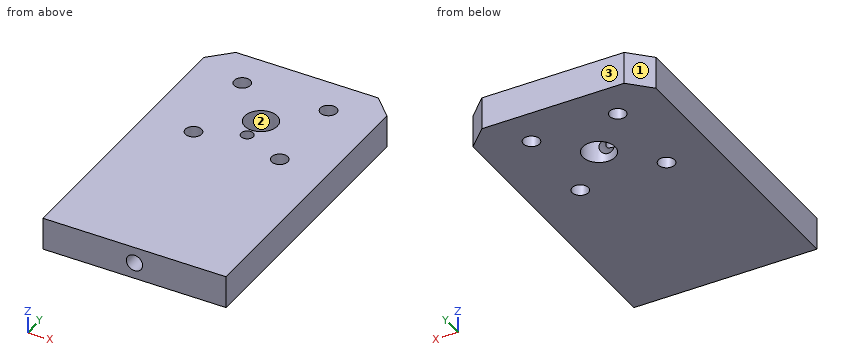
```python
from build123d import *

# Parameters (mm, degrees)
F0_R     = 2
F0_R_2   = 4
F1_DEPTH = 8
F2_R     = 2
F3_DEPTH = 53
F4_R     = 1.5
F5_DEPTH = 3


with BuildPart() as f1:
    # F0 (on Top) → F1 (new body)
    with BuildSketch(Plane.XY):
        Polygon((0, 70), (0, 0), (45, 0), (45, 70), (40, 75), (5, 75), align=None)
        with Locations((11.893398, 44.393398)):
            Circle(F0_R, mode=Mode.SUBTRACT)
        with Locations((11.893398, 65.606602)):
            Circle(F0_R, mode=Mode.SUBTRACT)
        with Locations((33.106602, 44.393398)):
            Circle(F0_R, mode=Mode.SUBTRACT)
        with Locations((22.5, 55)):
            Circle(F0_R_2, mode=Mode.SUBTRACT)
        with Locations((33.106602, 65.606602)):
            Circle(F0_R, mode=Mode.SUBTRACT)
    extrude(amount=F1_DEPTH)

    # F2 (on face) → F3 (cut)
    with BuildSketch(Plane.XZ):
        with Locations((22.5, 4)):
            Circle(F2_R)
    extrude(amount=-F3_DEPTH, mode=Mode.SUBTRACT)

    # F4 (on face) → F5 (cut)
    with BuildSketch(Plane.XY.offset(8)):
        with Locations((22.5, 49)):
            Circle(F4_R)
    extrude(amount=-F5_DEPTH, mode=Mode.SUBTRACT)


solid = f1.part
```
Work out the finished part from the listing and answer in its coordinate system (mm). Face numbers are marked on the shaded views. Give positions to 0.01 mm unless a question says otherwise; leave off trailing zeros. Loops run counter-clockwise (first coordinate to the right, second up) from the corner with the lowest first, then second, coordinate; pieces in that order, holes last. Notation, with made-up numbers: (41, -25.75) -> (74, -25.75) arc R21 cw to (74, 0.25) -> close; hole circle Ø4 at (-30.5, 34). An arc over 180 degrees is marked (long way). One line per question, with ' | ' between items. Start each with the question number.
1) Section B-B, the plane y = 32.5 is taken. Determine the outline of the cut face in (x, z).
2) Straight lines are drawn through the part: L1, parallel to Y at x = 33, z = 7.5; L2, parallel to Z at x = 22.5, y = 38.5; L3, parallel to X at y = 65, z = 2.5. For each, find the intervals that lie inside material, in ascending order.
3) This flat-tipped pin is pushed along its axis until it touches: pin 1 (3.5 mm diameter, centred on x = 33.11, y = 44.39, fed in from -Z). Where does it stop, or does it pass through?
4) Section A-A, the plane x = 22.5 is taken. Determine the outline of the cut face in (y, z), then the cut area to 3 significant figures.
5) Section C-C, the plane y = 55 is taken. Determine the outline of the cut face in (x, z), then the cut area to 3 significant figures.
6) Determine the mould class of the marked faces 1, 2 and 3 for opening direction X: +X half, -X half, draft (parallel to the pull), parting line (faces both ways), or undercut.
7) Section D-D, the plane z = 4 is taken. Determine the outline of the cut face in (x, y).
Resolved:
1) outline: (0, 0) -> (45, 0) -> (45, 8) -> (0, 8) -> close; hole circle Ø4 at (22.5, 4)
2) L1: 0 to 42.4, 46.39 to 63.61, 67.6 to 75 | L2: 0 to 2, 6 to 8 | L3: 0 to 9.99, 13.8 to 31.2, 35.01 to 45
3) pin 1: through
4) outline: (0, 0) -> (51, 0) -> (51, 2) -> (0, 2) -> close; (0, 6) -> (47.5, 6) -> (47.5, 8) -> (0, 8) -> close; (50.5, 6) -> (51, 6) -> (51, 8) -> (50.5, 8) -> close; (59, 0) -> (75, 0) -> (75, 8) -> (59, 8) -> close | area: 326 mm2
5) outline: (0, 0) -> (18.5, 0) -> (18.5, 8) -> (0, 8) -> close; (26.5, 0) -> (45, 0) -> (45, 8) -> (26.5, 8) -> close | area: 296 mm2
6) face 1: -X half | face 2: undercut | face 3: draft
7) outline: (0, 0) -> (20.5, 0) -> (20.5, 51.54) arc R4 cw (long way) to (24.5, 51.54) -> (24.5, 0) -> (45, 0) -> (45, 70) -> (40, 75) -> (5, 75) -> (0, 70) -> close; hole circle Ø4 at (11.89, 44.39); hole circle Ø4 at (11.89, 65.61); hole circle Ø4 at (33.11, 44.39); hole circle Ø4 at (33.11, 65.61)
